The listing builds one solid part. Answer for the finished solid, in the listing's coordinates (mm). A direction names the side the tool comes from. Round coordinates to 2 decimals unless told otherwise and drop trailing zeros. Write each loop counter-clockwise with the first axis right and the second up, starting at its lowest first coordinate (ties: lowest second). Pieces come first, ordered by that corner, then holes.
(1) Find the intervals of material crossed by probe 1 along Y at (x, z) = (0, 11); probe 2 along Y at (x, z) = (0, 2.6); probe 3 along Z at (x, y) = (6, -3), in increasing order.
(2) The mould has two halves that part along Y. Classify faces 1 (the face through (-0.16, 7.5, 2.83)), 2 (the face through (-7.5, -1, 9)), 3 (the face through (-2.75, -22, 1)): +Y half, -Y half, draft (parallel to the pull), parting line (faces both ways), or undercut.
(3) A cutting plane is placed at C-C, the plane y = 4.5. Give the vertices of the cut face in (x, z), and give its area (3 significant figures).
(4) A cutting plane is placed at B-B, the plane z = 4.25. Give the vertices of the cut face in (x, y), and give its area (3 significant figures).
(5) Each of these flat-tipped pins is pushed along its axis until it touches: pin 1 Ø8 at (x, z) = (0.5, 5) entering from +Y; pin 2 Ø6 at (y, z) = (2.5, 6.5) entering from -X; pin 3 Ø6 at (x, z) = (9.5, 14) entering from +Y; pin 4 Ø3 at (x, y) = (-0.5, -22) entering from -Z. Where does it stop, or does it pass through?
(6) A cutting plane is placed at D-D, the plane x = 11.5. Give the vertices of the cut face in (y, z).
(7) For faces 4 (the face through (-0.1, 6.5, 3.3)), 5 (the face through (-0.596, 2.685, 8.628)), 6 (the face through (0, -5, 17)), 7 (the face through (1, 7, 11.75)), 8 (the face through (0, -29, 1.25)), determine the directions among +Z, -Z, +X, -X, +Y, -Y from which every point of the face is accessible in a straight line to the end or side of a thin tool.
(8) A cutting plane is placed at A-A, the plane y = -22. Give the vertices of the cut face in (x, z).
Autodesk Inventor part; units mm, degrees
ref_plane "Work Plane2" through (0, -7.5, 0) normal (0, 1, 0) x (-1, 0, 0)
ref_plane "Work Plane3" through (0, 7.5, 0) normal (0, 1, 0) x (-1, 0, 0)
ref_plane "YZ Plane" through (0, 0, 0) normal (1, 0, 0) x (0, 1, 0)
sketch "Sketch1" plane through (0, 0, 0) normal (0, 0, 1) x (1, 0, 0)
  arc A0 (7.5, 0) -> (-7.5, 0) centre (0, 0) ccw
  line L0 (-7.5, 0) -> (-15, -20)
  line L1 (7.5, 0) -> (15, -20)
  line L2 (-7.5, 0) -> (7.5, 0) construction
  line L3 (-15, -30) -> (15, -30)
  line L4 (-15, -30) -> (15, -30) construction
  circle A1 centre (0, 0) radius 2.75
  line L5 (-15, -20) -> (-15, -30)
  line L6 (15, -20) -> (15, -30)
  dimension "d0" = 15
  dimension "d8" = 5.5
  dimension "d67" = 30
  dimension "d68" = 30
  dimension "d96" = 10
extrude "Extrusion1" add sketch "Sketch1" along normal blind 17.5
shell "Shell2" thickness 1 removed faces 1 at (0.1105, -14.2433, 17.5)
thicken "Thicken5" operation add thickness 2 both sides no extend neighbours no toward (0, 1, 0) faces at (-4.6667, -29, 6.5)
sketch "Sketch12" plane through (-15, -30, 0) normal (0, -1, 0) x (1, 0, 0)
  line L0 (0, 0) -> (30, 0)
  line L1 (30, 0) -> (30, 17.5)
  line L2 (0, 17.5) -> (30, 17.5)
  line L3 (0, 0) -> (0, 17.5)
  line L4 (25.5, 16.25) -> (4.5, 16.25)
  line L5 (4.5, 16.25) -> (4.5, 1.25)
  line L6 (4.5, 1.25) -> (25.5, 1.25)
  line L7 (25.5, 1.25) -> (25.5, 16.25)
  line L8 (25.5, 16.25) -> (25.5, 17.5)
  line L9 (21.4976, 17.5) -> (29, 17.5)
  line L10 (25.5, 1.25) -> (25.5, 0)
  line L11 (0, 0) -> (30, 0)
  point P0 (15, 0)
  dimension "d74" = 21
  dimension "d75" = 15
  dimension "d77" = 4.5
  dimension "d78" = 4.5
  dimension "d79" = 1.25
extrude "Extrusion6" cut sketch "Sketch12" against normal blind 2 contours L6 L5 L4 L7
sketch "Sketch13" plane through (-15, -28, 0) normal (0, -1, 0) x (1, 0, 0)
  line L0 (25.5, 16.25) -> (25.5, 1.25)
  line L1 (4.5, 1.25) -> (4.5, 16.25)
  line L2 (4.5, 13.75) -> (9.5, 13.75)
  line L3 (9.5, 13.75) -> (9.5, 3.75)
  line L4 (9.5, 3.75) -> (4.5, 3.75)
  line L5 (4.5, 3.75) -> (4.5, 13.75)
  line L6 (4.5, 16.25) -> (25.5, 16.25)
  line L7 (25.5, 1.25) -> (4.5, 1.25)
  line L8 (25.5, 13.75) -> (20.5, 13.75)
  line L9 (20.5, 13.75) -> (20.5, 3.75)
  line L10 (20.5, 3.75) -> (25.5, 3.75)
  line L11 (25.5, 3.75) -> (25.5, 13.75)
  point P0 (15, 0)
  dimension "d82" = 5
  dimension "d83" = 10
  dimension "d84" = 2.5
  dimension "d85" = 2.5
  dimension "d86" = 5
  dimension "d87" = 10
  dimension "d88" = 2.5
  dimension "d89" = 2.5
extrude "Extrusion7" cut sketch "Sketch13" against normal up to next contours L0 L10 L9 L8 | L2 L3 L4 L1
sketch "Sketch14" plane through (-15, -28, 0) normal (0, -1, 0) x (1, 0, 0)
  line L0 (4.5, 16.25) -> (25.5, 16.25)
  line L1 (25.5, 16.25) -> (25.5, 1.25)
  line L2 (4.5, 1.25) -> (4.5, 16.25)
  line L3 (25.5, 1.25) -> (4.5, 1.25)
  line L4 (15, 1.25) -> (15, 16.25) construction
  line L5 (25.5, 8.75) -> (4.5, 8.75) construction
  line L6 (4.5, 13.75) -> (4.5, 3.75)
  point P0 (15, 0)
  point P1 (15, 9.5)
ref_plane "Work Plane2" through (0, -7.5, 0) normal (0, 1, 0) x (-1, 0, 0)
sketch "Sketch16" plane through (0, 0, 1) normal (0, 0, 1) x (1, 0, 0)
  line L0 (14, -27) -> (-14, -27)
  line L1 (0, -27) -> (0, -16.6699) construction
  point P0 (0, 0)
  point P1 (0, -22)
  point P2 (-0.2812, -15.3392)
  point P3 (3.9903, -15.1005)
  dimension "d97" = 5
hole "Hole3" at (0, -22, 1) direction (0, 0, -1) diameter 3.4 depth 1
sketch "Sketch17" plane through (0, 0, 1) normal (0, 0, 1) x (1, 0, 0)
  circle A0 centre (0, -22) radius 1.7
  circle A1 centre (0, -22) radius 4.75
  point P0 (0, 0)
  dimension "d105" = 9.5
extrude "Extrusion9" add sketch "Sketch17" along normal blind 2
sketch "Sketch18" plane through (0, 0, 0) normal (0, 0, -1) x (-1, 0, 0)
  circle A0 centre (0, -22) radius 1.7
  circle A1 centre (0, -22) radius 2.75 construction
  line L0 (2.75, -20.4123) -> (2.75, -23.5877)
  line L1 (2.75, -23.5877) -> (0, -25.1754)
  line L2 (0, -25.1754) -> (-2.75, -23.5877)
  line L3 (-2.75, -23.5877) -> (-2.75, -20.4123)
  line L4 (-2.75, -20.4123) -> (0, -18.8246)
  line L5 (0, -18.8246) -> (2.75, -20.4123)
  point P0 (0, 0)
  dimension "d108" = 5.5
extrude "Extrusion10" cut sketch "Sketch18" against normal blind 2
ref_plane "Work Plane3" through (0, 7.5, 0) normal (0, 1, 0) x (-1, 0, 0)
sketch "Sketch19" plane through (0, 7.5, 0) normal (0, 1, 0) x (-1, 0, 0)
  line L0 (-14, 17.5) -> (14, 17.5)
  line L1 (0, 17.5) -> (0, 0) construction
  line L2 (-7.5, 11.75) -> (7.5, 11.75)
  line L3 (7.5, 11.75) -> (7.5, 5.75)
  line L4 (7.5, 5.75) -> (-7.5, 5.75)
  line L5 (-7.5, 5.75) -> (-7.5, 11.75)
  line L6 (-7.5, 11.75) -> (7.5, 5.75) construction
  line L7 (7.5, 11.75) -> (-7.5, 5.75) construction
  point P0 (0, 8.75)
  dimension "d111" = 15
  dimension "d112" = 6
extrude "Extrusion11" cut sketch "Sketch19" against normal up to next
sketch "Sketch22" plane through (0, 0, 17.5) normal (0, 0, 1) x (1, 0, 0)
  line L0 (-8.307, -5) -> (8.307, -5)
  line L1 (6.4976, -0.175) -> (14, -20.1813)
  line L2 (-14, -20.1813) -> (-6.4976, -0.175)
  arc A0 (6.4976, -0.175) -> (-6.4976, -0.175) centre (0, 0) ccw
  circle A1 centre (0, 0) radius 2.75
  dimension "d117" = 5
extrude "Extrusion13" add sketch "Sketch22" against normal blind 2
properties part number "LampeSolaire2_LedAmoviblePart 3D printed"
Solutions:
1. probe 1: y = -28 to -27, -3.75 to -2.75, 2.75 to 3.75
1. probe 2: y = -28 to -27, -26.75 to -23.7, -20.3 to -17.25, -3.75 to -2.75, 2.75 to 3.75, 6.5 to 7.5
1. probe 3: z = 0 to 1, 15.5 to 17.5
2. face 1: +Y half
2. face 2: draft
2. face 3: undercut
3. outline: (-6, 0) - (6, 0) - (6, 5.75) - (4.69, 5.75) - (4.69, 1) - (-4.69, 1) - (-4.69, 5.75) - (-6, 5.75) - close; (-6, 11.75) - (-4.69, 11.75) - (-4.69, 15.5) - (4.69, 15.5) - (4.69, 11.75) - (6, 11.75) - (6, 17.5) - (-6, 17.5) - close
3. area: 58.3 mm2
4. outline: (-15, -30) - (-10.5, -30) - (-10.5, -27) - (-14, -27) - (-14, -20.18) - (-6.5, -0.18) arc R6.5 cw (long way) to (6.5, -0.18) - (14, -20.18) - (14, -27) - (10.5, -27) - (10.5, -30) - (15, -30) - (15, -20) - (7.5, 0) arc R7.5 ccw to (-7.5, 0) - (-15, -20) - close; (-5.5, -28) - (5.5, -28) - (5.5, -27) - (-5.5, -27) - close; circle Ø7.5 at (0, 0); hole circle Ø5.5 at (0, 0)
4. area: 137 mm2
5. pin 1: stops at y = 7.5
5. pin 2: stops at x = -7.69
5. pin 3: stops at y = 3.74
5. pin 4: stops at z = 2
6. outline: (-30, 0) - (-10.67, 0) - (-10.67, 17.5) - (-13.51, 17.5) - (-13.51, 1) - (-27, 1) - (-27, 17.5) - (-30, 17.5) - close
7. face 4: none
7. face 5: +Z, -Z
7. face 6: +Z
7. face 7: +Y
7. face 8: -Y
8. outline: (-15, 0) - (-2.75, 0) - (-2.75, 2) - (-1.7, 2) - (-1.7, 3) - (-4.75, 3) - (-4.75, 1) - (-14, 1) - (-14, 17.5) - (-15, 17.5) - close; (1.7, 2) - (2.75, 2) - (2.75, 0) - (15, 0) - (15, 17.5) - (14, 17.5) - (14, 1) - (4.75, 1) - (4.75, 3) - (1.7, 3) - close
